Autodesk Inventor part; units mm, degrees
ref_plane "YZ Plane" through (0, 0, 0) normal (1, 0, 0) x (0, 1, 0)
ref_plane "XZ Plane" through (0, 0, 0) normal (0, 1, 0) x (-1, 0, 0)
ref_plane "XY Plane" through (0, 0, 0) normal (0, 0, 1) x (1, 0, 0)
sketch "Sketch1" plane through (0, 0, 0) normal (0, 1, 0) x (-1, 0, 0)
  circle A0 centre (0, 0) radius 22.75
  circle A1 centre (0, 0) radius 52
  circle A2 centre (0, 0) radius 27.75
  dimension "d0" = 45.5
  dimension "d1" = 104
  dimension "d2" = 55.5
extrude "Extrusion1" add sketch "Sketch1" along normal blind 7 contours A1 | A2
extrude "Extrusion2" add sketch "Sketch1" against normal blind 5.75 contours A2
fillet "Fillet1" radius 5 1 edges at (52, 0, 0)
properties part number "motor_chain_guide_outer"
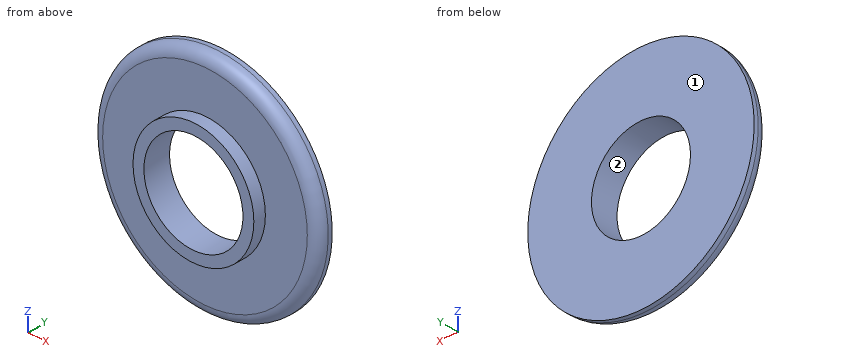
Source: CAD feature listing. Evaluate the final solid. Frame: model axes, mm. Face numbers are marked on the shaded views. Give positions to 0.01 mm unless a question says otherwise; leave off trailing zeros. Loops run counter-clockwise (first coordinate to the right, second up) from the corner with the lowest first, then second, coordinate; pieces in that order, holes last. Notation, with made-up numbers: M -30,-13.75 L 8,-13.75 A10 ccw 8,2.25 Z; hole C 9,-34.5 d5. An arc over 180 degrees is marked long. Put each result on its own line as item: value.
Q1. Mould query, pull axis Z, two halves, no side actions, for the marked faces 1 and 2. Classes: released by +Z, released by -Z, zero draft, split by the parting line, or undercut.
Response values:
face 1: zero draft
face 2: undercut
Q2. Section B-B (x = 0). Return the cut outline in (y, z), and give its area (3 significant figures).
Response values:
outline: M -5.75,-27.75 L 0,-27.75 L 0,-47 A5 ccw 5,-52 L 7,-52 L 7,-22.75 L -5.75,-22.75 Z; M -5.75,22.75 L 7,22.75 L 7,52 L 5,52 A5 ccw 0,47 L 0,27.75 L -5.75,27.75 Z
area: 456 mm²
Q3. Pin query (flat end, axial travel): P1, Ø1.5, axis at x = -36.5, z = -13.5, coming from the -Y side; P2, Ø3, axis at y = 1, z = 32, coming from the +X side; P3, Ø6, axis at x = 8.5, y = -3.5, coming from the +Z side. Return the tip coordinate at first contact, or that it passes through.
Response values:
P1: stops at y = 0
P2: stops at x = 40.61
P3: stops at z = 27.2
Q4. Section C-C (y = -1.75). Return the cut outline in (x, z).
Response values:
outline: C 0,0 d55.5; hole C 0,0 d45.5
Q5. Line query: probe 1 along Z at (x, y) = (0, -0.5); probe 2 along Y at (x, z) = (-33, 13); probe 3 along X at (y, z) = (4.5, -19). Output: solid intervals per line, ascending. Write a range as [from, to].
Response values:
probe 1: z = [-27.75, -22.75], [22.75, 27.75]
probe 2: y = [0, 7]
probe 3: x = [-48.38, -12.51], [12.51, 48.38]
Q6. Section A-A (z = 0). Return the cut outline in (x, y), and give its area (3 significant figures).
Response values:
outline: M -52,5 A5 ccw -47,0 L -27.75,0 L -27.75,-5.75 L -22.75,-5.75 L -22.75,7 L -52,7 Z; M 22.75,-5.75 L 27.75,-5.75 L 27.75,0 L 47,0 A5 ccw 52,5 L 52,7 L 22.75,7 Z
area: 456 mm²
